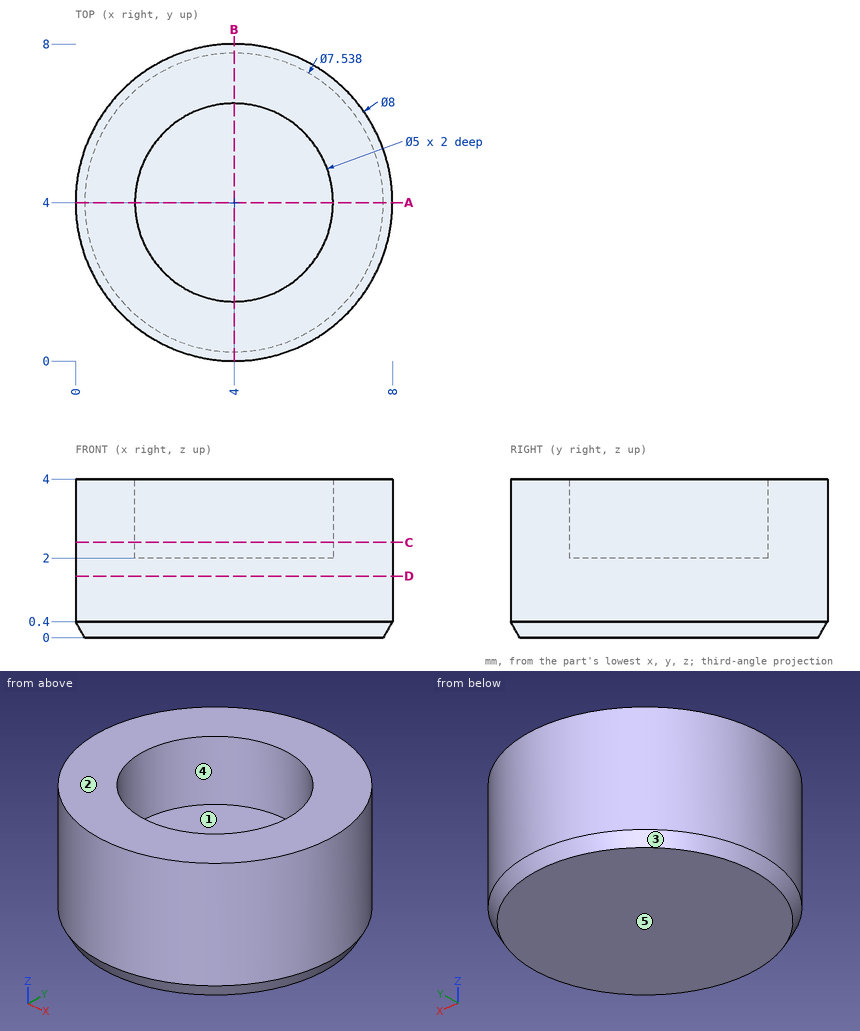
Input: dimensioned drawing with shaded views. Units: mm. Origin: part minimum x, y, z. A direction names the side the tool comes from. Coordinates: 2 decimals unless noted, no trailing zeros. Write each loop counter-clockwise with the first axis right and the second up, starting at its lowest first coordinate (ties: lowest second). Pieces come first, ordered by that corner, then holes. Notation, with made-up numbers: M 2,18.25 L 34,18.25 A25 cw 34,49.25 Z; hole C 39.25,46 d2. An arc over 180 degrees is marked long. Answer as a JSON object with one key per item and string values. Group by question number.
(1) Contact query for flat-ended pins moving along their axis: P1, Ø1, axis at y = 2, z = 3.5, coming from the +X side; P2, Ø1.5, axis at x = 5.5, z = 1, coming from the +Y side; P3, Ø3, axis at x = 3.5, y = 3.5, coming from the +Z side. Output: stop coordinate, or through.
(2) Mould query, pull axis Y, two halves, no side actions, for the marked faces 1, 2 and 3. Classes: pulls with the +Y half, pulls with the -Y half, needs draft (parallel to the pull), parting line crosses it, or undercut.
(3) Ray query, line 1 along Y through (x, z) = (4, 2.6); line 2 along Z through (x, y) = (4, 4); line 3 along X through (y, z) = (6, 3.25) (1 decimal). Return the intervals inside material, ascending. Write a range as [from, to].
(4) Set-up query: the marked faces 4 and 5. Return all of +Z, -Z, +X, -X, +Y, -Y with unobstructed straight access to the full face (end or side cutting, diameter ignored); none if empty.
(5) Section C-C on z = 2.4. Output: boundary loops of the cut face in (x, y).
(6) Section A-A on y = 4. Output: boundary loops of the cut face in (x, z), plus the area to 3 significant figures.
(7) Section D-D on z = 1.55. Output: boundary loops of the cut face in (x, y).
Result set:
{
 "1": {"P1": "stops at x = 7.71", "P2": "stops at y = 7.93", "P3": "stops at z = 2"},
 "2": {"face 1": "undercut", "face 2": "needs draft", "face 3": "parting line crosses it"},
 "3": {"line 1": "y = [0, 1.5], [6.5, 8]", "line 2": "z = [0, 2]", "line 3": "x = [0.5, 2.5], [5.5, 7.5]"},
 "4": {"face 4": "+Z", "face 5": "-Z, +X, -X, +Y, -Y"},
 "5": {"outline": "C 4,4 d8; hole C 4,4 d5"},
 "6": {"outline": "M 0,0.4 L 0.23,0 L 7.77,0 L 8,0.4 L 8,4 L 6.5,4 L 6.5,2 L 1.5,2 L 1.5,4 L 0,4 Z", "area": "21.9 mm2"},
 "7": {"outline": "C 4,4 d8"}
}
